Design review of the part built by this model. Coordinates are the model's own, in mm. Round coordinates to 2 decimals unless told otherwise and drop trailing zeros. Loops run counter-clockwise (first coordinate to the right, second up) from the corner with the lowest first, then second, coordinate; pieces in that order, holes last. Notation, with made-up numbers: (25.5, -19.75) - (58.5, -19.75) arc R20 cw to (58.5, 16.25) - close; hole circle Ø9 at (-23.75, 56). An arc over 180 degrees is marked (long way). Use one line per item in the form item = value. Start each with the question number.
(1) We need section A-A, the plane x = 57. Write out the cut boundary in (y, z).
(2) We need section B-B, the plane z = 0. Write out the cut boundary in (x, y).
(3) For pin 1 (2 mm diameter, centred on y = 15, z = -1, fed in from -X); pin 2 (1.5 mm diameter, centred on y = 58.5, z = -3, fed in from +X), all flat-tipped, find the tip position at first contact; note any pin that passes through.
(4) We need section C-C, the plane y = 27. Write out the cut boundary in (x, z).
(5) Wall thickness on probe 1 along Y at (x, z) = (93.5, -0.25); probe 2 along X at (y, z) = (1.3, 0); probe 3 along X at (y, z) = (50.5, 0): over which ranges is each line inside the solid? List them lowest first. Write a range as [from, to].
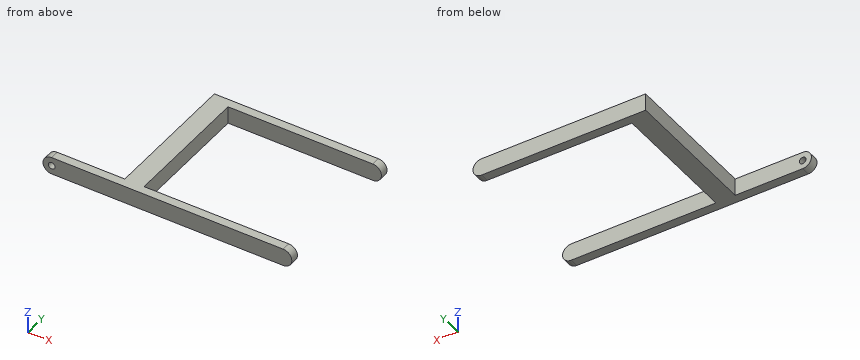
from build123d import *

# Parameters (mm, degrees)
BOSS_EXTRUDE1_DEPTH = 4.5
SKETCH2_R           = 1.75
CUT_EXTRUDE1_DEPTH  = 10
SKETCH3_W           = 10
SKETCH3_H           = 9
BOSS_EXTRUDE2_DEPTH = 67.5
SKETCH4_W           = 85
SKETCH4_H           = 9
BOSS_EXTRUDE3_DEPTH = 4.5
BOSS_EXTRUDE4_START = -4.5
SKETCH5_R           = 4.5
BOSS_EXTRUDE4_DEPTH = 4.5


with BuildPart() as part:
    # Sketch1 → Boss-Extrude1 (new body)
    with BuildSketch(Plane(origin=(0, 0, 0), x_dir=(1, 0, 0), z_dir=(0, 1, 0))):
        with BuildLine():
            Line((0, 4.5), (120, 4.5))
            ThreePointArc((120, 4.5), (124.5, 0), (120, -4.5))
            Line((120, -4.5), (0, -4.5))
            ThreePointArc((0, -4.5), (-4.5, 0), (0, 4.5))
        make_face()
    extrude(amount=BOSS_EXTRUDE1_DEPTH)

    # Sketch2 → Cut-Extrude1 (cut)
    with BuildSketch(Plane(origin=(0, 4.5, 0), x_dir=(1, 0, 0), z_dir=(0, 1, 0))):
        with Locations(Location((0, 0, 0), (0, 0, 270))):
            Circle(SKETCH2_R)
    extrude(amount=-CUT_EXTRUDE1_DEPTH, mode=Mode.SUBTRACT)

    # Sketch3 → Boss-Extrude2 (add)
    with BuildSketch(Plane(origin=(0, 4.5, 0), x_dir=(1, 0, 0), z_dir=(0, 1, 0))):
        with Locations((40, 0)):
            Rectangle(SKETCH3_W, SKETCH3_H)
    extrude(amount=BOSS_EXTRUDE2_DEPTH)

    # Sketch4 → Boss-Extrude3 (add)
    with BuildSketch(Plane(origin=(0, 72, 0), x_dir=(1, 0, 0), z_dir=(0, 1, 0))):
        with Locations((77.5, 0)):
            Rectangle(SKETCH4_W, SKETCH4_H)
    extrude(amount=BOSS_EXTRUDE3_DEPTH)

    # Sketch5 → Boss-Extrude4 (add)
    with BuildSketch(Plane(origin=(0, 76.5, 0), x_dir=(1, 0, 0), z_dir=(0, 1, 0)).offset(BOSS_EXTRUDE4_START)):
        with Locations((120, 0)):
            Circle(SKETCH5_R)
    extrude(amount=BOSS_EXTRUDE4_DEPTH)


solid = part.part
Data:
q1.outline = (0, -4.5) - (4.5, -4.5) - (4.5, 4.5) - (0, 4.5) - close; (72, -4.5) - (76.5, -4.5) - (76.5, 4.5) - (72, 4.5) - close
q2.outline = (-4.5, 0) - (-1.75, 0) - (-1.75, 4.5) - (-4.5, 4.5) - close; (1.75, 0) - (124.5, 0) - (124.5, 4.5) - (45, 4.5) - (45, 72) - (124.5, 72) - (124.5, 76.5) - (35, 76.5) - (35, 4.5) - (1.75, 4.5) - close
q3.pin_1 = 35
q3.pin_2 = 45
q4.outline = (35, -4.5) - (45, -4.5) - (45, 4.5) - (35, 4.5) - close
q5.probe_1 = [0, 4.5], [72, 76.5]
q5.probe_2 = [-4.5, -1.75], [1.75, 124.5]
q5.probe_3 = [35, 45]
